For this review, use the dimensioned drawing (mm, ordinates from the lowest corner) and the shaded views. Coordinates: 2 decimals unless noted, no trailing zeros. Loops run counter-clockwise (first coordinate to the right, second up) from the corner with the lowest first, then second, coordinate; pieces in that order, holes last. Notation, with made-up numbers: (-17, -38) - (33, -38) arc R24 ccw to (33, 1) - close; hole circle Ø8 at (89, 70). An arc over 180 degrees is marked (long way). Answer in a Markdown table with one row per item. Add a question column.
(1) To check wall thickness, follow L1, parallel to X at y = 0.4, z = 10; L2, parallel to X at y = 3, z = 10; L3, parallel to Y at x = 5, z = 6.5. State the ranges of each line that lie inside material, in increasing order. Write a range as [from, to].
(2) The part is to be moulded in two halves that separate along Z. For the marked faces 1, 2 and 3, say which applies: released by +Z, released by -Z, zero draft, split by the parting line, or undercut.
(3) We need section D-D, the plane y = 1.25. Write out the cut boundary in (x, z).
(4) We need section C-C, the plane x = 5.25. Write out the cut boundary in (y, z).
(5) Clearance check with flat-ended pins moving along their axes: pin 1 (2 mm diameter, centred on y = 1, z = 12, fed in from -X); pin 2 (1.5 mm diameter, centred on x = 5.5, y = 2.5, fed in from -Z); pin 3 (1.5 mm diameter, centred on y = 2.5, z = 7.5, fed in from +X). State where each tip first meets the part, or that it passes through.
(6) We need section B-B, the plane x = 10. Write out the cut boundary in (y, z).
(7) We need section A-A, the plane z = 10. Write out the cut boundary in (x, y), plus the area to 3 significant figures.
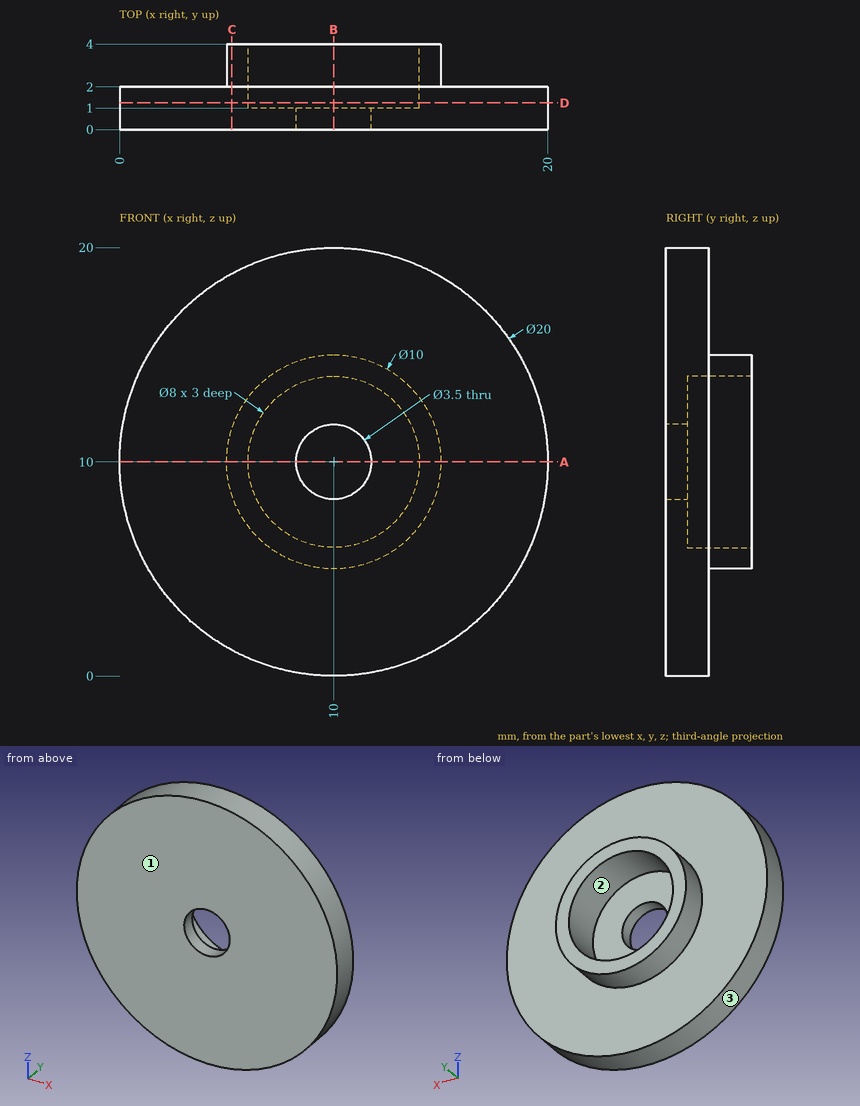
Responses:
| question | item | result |
|---|---|---|
| 1 | L1 | x = [0, 8.25], [11.75, 20] |
| 1 | L2 | x = [5, 6], [14, 15] |
| 1 | L3 | y = [0, 2] |
| 2 | face 1 | zero draft |
| 2 | face 2 | undercut |
| 2 | face 3 | split by the parting line |
| 3 | outline | circle Ø20 at (10, 10); hole circle Ø8 at (10, 10) |
| 4 | outline | (0, 1.2) - (2, 1.2) - (2, 8.44) - (4, 8.44) - (4, 11.56) - (2, 11.56) - (2, 18.8) - (0, 18.8) - close |
| 5 | pin 1 | stops at x = 0.05 |
| 5 | pin 2 | stops at z = 0.81 |
| 5 | pin 3 | stops at x = 19.81 |
| 6 | outline | (0, 0) - (2, 0) - (2, 5) - (4, 5) - (4, 6) - (1, 6) - (1, 8.25) - (0, 8.25) - close; (0, 11.75) - (1, 11.75) - (1, 14) - (4, 14) - (4, 15) - (2, 15) - (2, 20) - (0, 20) - close |
| 7 | outline | (0, 0) - (8.25, 0) - (8.25, 1) - (6, 1) - (6, 4) - (5, 4) - (5, 2) - (0, 2) - close; (11.75, 0) - (20, 0) - (20, 2) - (15, 2) - (15, 4) - (14, 4) - (14, 1) - (11.75, 1) - close |
| 7 | area | 32.5 mm2 |
